The figure shows three views and two pictorial views of one solid part (mm, origin at its lowest corner). Answer the questions. Round coordinates to 2 decimals unless told otherwise and drop trailing zeros. Write each loop counter-clockwise with the first axis right and the second up, starting at its lowest first coordinate (ties: lowest second). Pieces come first, ordered by that corner, then holes. Notation, with made-up numbers: M -14.5,-9.5 L 4.5,-9.5 A11 ccw 4.5,5.5 Z; hole C -7,17 d3. An arc over 180 degrees is marked long. One line per item, written item: value. Start each with the question number.
Q1. Given pin 1 Ø1.7 at (x, y) = (127, 20.6) entering from -Z; pin 2 Ø0.9 at (y, z) = (20, 1) entering from -X, each flat-ended and moving along its own axis, determine where each tip first touches the part or whether it passes through.
Q2. Consider probe 1 along Y at (x, z) = (127, 1.2); probe 2 along Y at (x, z) = (40, 2.8); probe 3 along X at (y, z) = (5, 2.25). Determine where each line is inside the solid, lowest interval first.
Q3. Find section B-B (z = 1.6). Write down the section's boundary in (x, y).
Q4. Find section A-A (x = 13). Write down the section's boundary in (y, z).
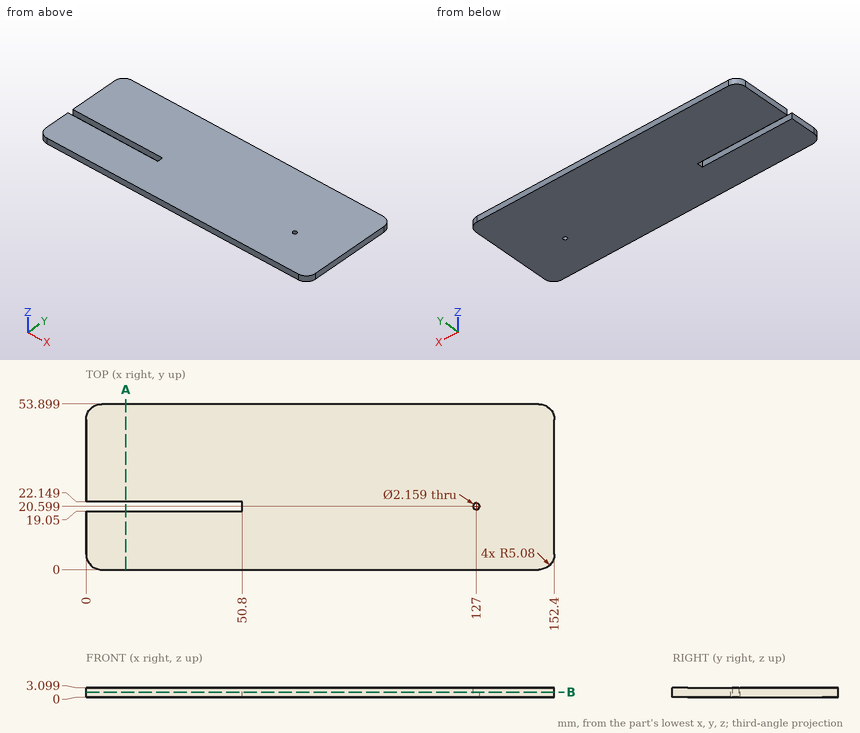
The answers:
1. pin 1: through
1. pin 2: x = 50.8
2. probe 1: 0 to 19.52, 21.68 to 53.9
2. probe 2: 0 to 19.05, 22.15 to 53.9
2. probe 3: 0 to 152.4
3. outline: M 0,5.08 A5.08 ccw 5.08,0 L 147.32,0 A5.08 ccw 152.4,5.08 L 152.4,48.82 A5.08 ccw 147.32,53.9 L 5.08,53.9 A5.08 ccw 0,48.82 L 0,22.15 L 50.8,22.15 L 50.8,19.05 L 0,19.05 Z; hole C 127,20.6 d2.16
4. outline: M 0,0 L 19.05,0 L 19.05,3.1 L 0,3.1 Z; M 22.15,0 L 53.9,0 L 53.9,3.1 L 22.15,3.1 Z
